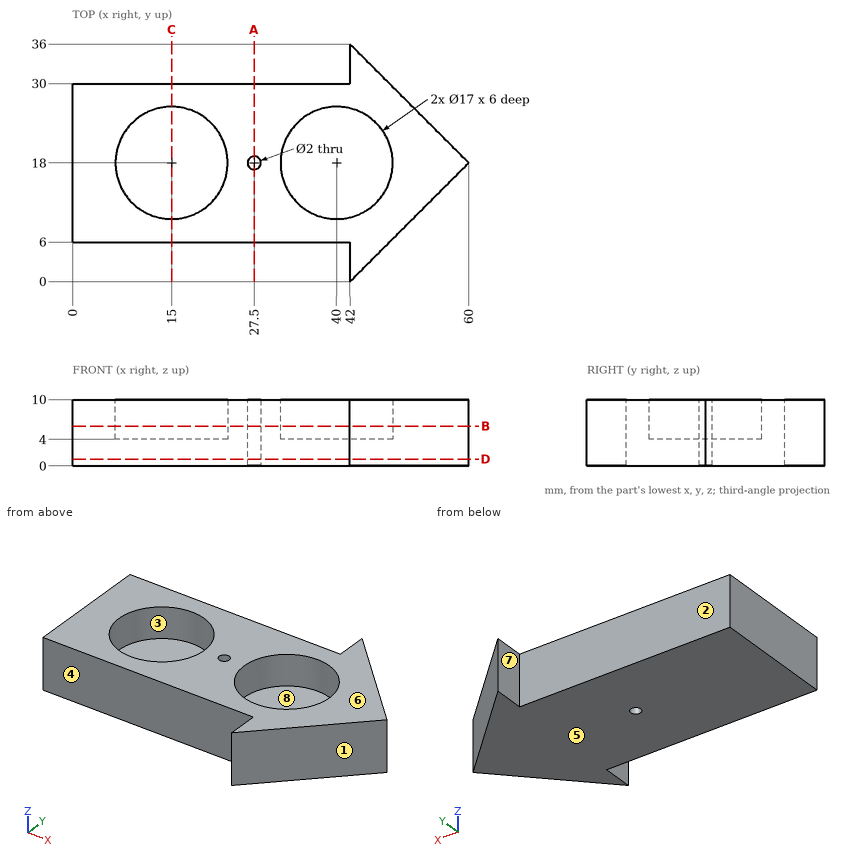
Answer from the drawing. Dimensions are ordinates in mm from the lowest x, y and z of the part. A direction names the side the tool comes from. Round coordinates to 2 decimals unless told otherwise and drop trailing zeros. Write each loop counter-clockwise with the first axis right and the second up, starting at its lowest first coordinate (ties: lowest second). Pieces come first, ordered by that corner, then holes.
1. The part is cut by section A-A, the plane x = 27.5. Determine the outline of the cut face in (y, z).
2. Straight lines are drawn through the part: L1, parallel to Y at x = 27.5, z = 3; L2, parallel to X at y = 25, z = 4.25; L3, parallel to Y at x = 24, z = 2.25. For each, find the intervals that lie inside material, in ascending order.
3. The part is cut by section C-C, the plane x = 15. Determine the outline of the cut face in (y, z).
4. Given pin 1 Ø5 at (y, z) = (2, 4) entering from -X; pin 2 Ø3 at (x, z) = (34.5, 1.5) entering from +Y; pin 3 Ø3 at (y, z) = (29, 7.5) entering from +X, each flat-ended and moving along its own axis, determine where each tip first touches the part or whether it passes through.
5. The part is cut by section B-B, the plane z = 6. Determine the outline of the cut face in (x, y).
6. The part is cut by section D-D, the plane z = 1. Determine the outline of the cut face in (x, y), then the cut area to 3 significant figures.
7. Determine the mould class of the marked faces 6, 7 and 8 for opening direction X: pulls with the +X half, pulls with the -X half, needs draft (parallel to the pull), parting line crosses it, or undercut.
8. Which of the six approach directions +Z, -Z, +X, -X, +Y, -Y give full straight-line access (tool end or side, diameter ignored) to the marked faces 1, 2, 3, 4 and 5?
Values:
1. outline: (6, 0) - (17, 0) - (17, 10) - (6, 10) - close; (19, 0) - (30, 0) - (30, 10) - (19, 10) - close
2. L1: y = 6 to 17, 19 to 30
2. L2: x = 0 to 10.18, 19.82 to 35.18, 44.82 to 53
2. L3: y = 6 to 30
3. outline: (6, 0) - (30, 0) - (30, 10) - (26.5, 10) - (26.5, 4) - (9.5, 4) - (9.5, 10) - (6, 10) - close
4. pin 1: stops at x = 42
4. pin 2: stops at y = 30
4. pin 3: stops at x = 50.5
5. outline: (0, 6) - (42, 6) - (42, 0) - (60, 18) - (42, 36) - (42, 30) - (0, 30) - close; hole circle Ø17 at (15, 18); hole circle Ø2 at (27.5, 18); hole circle Ø17 at (40, 18)
6. outline: (0, 6) - (42, 6) - (42, 0) - (60, 18) - (42, 36) - (42, 30) - (0, 30) - close; hole circle Ø2 at (27.5, 18)
6. area: 1,330 mm2
7. face 6: needs draft
7. face 7: pulls with the -X half
7. face 8: undercut
8. face 1: +Z, -Z, +X, -Y
8. face 2: +Z, -Z, -X, +Y
8. face 3: +Z
8. face 4: +Z, -Z, -X, -Y
8. face 5: -Z, +X, -X, +Y, -Y
